from build123d import *

# Parameters (mm, degrees)
BOX001_W          = 10
BOX001_H          = 10
BOX001_DEPTH      = 8
CYLINDER_R        = 2.7
CYLINDER_DEPTH    = 10
CYLINDER001_R     = 3.5
CYLINDER001_DEPTH = 10
BOX_W             = 16
BOX_H             = 16
BOX_DEPTH         = 10


with BuildPart() as cube001:
    # Box001 → Box001 (new body)
    with BuildSketch(Plane(origin=(-5, -5, 0), x_dir=(1, 0, 0), z_dir=(0, 0, 1))):
        with Locations((5, 5)):
            Rectangle(BOX001_W, BOX001_H)
    extrude(amount=BOX001_DEPTH)


with BuildPart() as cylinder:
    # Cylinder → Cylinder (new body)
    with BuildSketch(Plane.XY.offset(10)):
        Circle(CYLINDER_R)
    extrude(amount=CYLINDER_DEPTH)


with BuildPart() as cut:
    # Cylinder001 → Cylinder001 (new body)
    with BuildSketch(Plane.XY.offset(10)):
        Circle(CYLINDER001_R)
    extrude(amount=CYLINDER001_DEPTH)

    # Cut: cut Cylinder
    add(cylinder.part, mode=Mode.SUBTRACT)


with BuildPart() as cut001:
    # Box → Box (new body)
    with BuildSketch(Plane(origin=(-8, -8, 0), x_dir=(1, 0, 0), z_dir=(0, 0, 1))):
        with Locations((8, 8)):
            Rectangle(BOX_W, BOX_H)
    extrude(amount=BOX_DEPTH)

    # Fusion: union Cut
    add(cut.part)

    # Cut001: cut Cube001
    add(cube001.part, mode=Mode.SUBTRACT)


solid = cut001.part
The model under review builds one solid part; all positions refer to its coordinate system, in mm. A direction names the side the tool comes from. Round coordinates to 2 decimals unless told otherwise and drop trailing zeros. Loops run counter-clockwise (first coordinate to the right, second up) from the corner with the lowest first, then second, coordinate; pieces in that order, holes last. Notation, with made-up numbers: (-14, 72) -> (41, 72) arc R17 cw to (41, 97) -> close; hole circle Ø9 at (44, 12.25). An arc over 180 degrees is marked (long way). Return JSON: item names as keys, results as strings.
(1) Add section B-B on x = 0. Write out the cut boundary in (y, z).
Solved:
{"outline": "(-8, 0) -> (-5, 0) -> (-5, 8) -> (5, 8) -> (5, 0) -> (8, 0) -> (8, 10) -> (3.5, 10) -> (3.5, 20) -> (2.7, 20) -> (2.7, 10) -> (-2.7, 10) -> (-2.7, 20) -> (-3.5, 20) -> (-3.5, 10) -> (-8, 10) -> close"}
(2) For faces 1 (the flat face through (-0.1, 5.4, 0)), 2 (the flat face through (-5, 0, 4)), 3 (the flat face through (-4, 0, 10)), list the 3-axis set-ups (+Z, -Z, +X, -X, +Y, -Y) from which the entire face can be reached by the end or side of a thin tool; tool diameter is ignored.
Solved:
{"face 1": "-Z, +X, -X, +Y, -Y", "face 2": "-Z", "face 3": "+Z"}
(3) Add section D-D on x = -3. Write out the cut boundary in (y, z), plus the area to 3 significant figures.
Solved:
{"outline": "(-8, 0) -> (-5, 0) -> (-5, 8) -> (5, 8) -> (5, 0) -> (8, 0) -> (8, 10) -> (1.8, 10) -> (1.8, 20) -> (-1.8, 20) -> (-1.8, 10) -> (-8, 10) -> close", "area": "116 mm2"}
(4) Add section C-C on y = -2. Write out the cut boundary in (x, z), plus the area to 3 significant figures.
Solved:
{"outline": "(-8, 0) -> (-5, 0) -> (-5, 8) -> (5, 8) -> (5, 0) -> (8, 0) -> (8, 10) -> (2.87, 10) -> (2.87, 20) -> (1.81, 20) -> (1.81, 10) -> (-1.81, 10) -> (-1.81, 20) -> (-2.87, 20) -> (-2.87, 10) -> (-8, 10) -> close", "area": "101 mm2"}
(5) For line 1 (X direction, y = 0.25, z = 1); line 2 (Y direction, x = 0, z = 12.25), list the stretches that pass through material, from the lowest coordinate up.
Solved:
{"line 1": "-8 to -5, 5 to 8", "line 2": "-3.5 to -2.7, 2.7 to 3.5"}
(6) The part is to be moulded in two halves that separate along Y. For faces 4 (the flat face through (0, -8, 5)), 5 (the flat face through (-8, 0, 5)), 6 (the flat face through (0, 5, 4)), say which applies: released by +Y, released by -Y, zero draft, split by the parting line, or undercut.
Solved:
{"face 4": "released by -Y", "face 5": "zero draft", "face 6": "undercut"}
(7) For pin 1 (4.5 mm diameter, centred on x = 0, y = 0, fed in from -Z); pin 2 (1.6 mm diameter, centred on x = 0, y = 0.5, fed in from +Z); pin 3 (3 mm diameter, centred on x = 3.5, z = 14, fed in from +Y), all flat-tipped, find the tip position at first contact; note any pin that passes through.
Solved:
{"pin 1": "z = 8", "pin 2": "z = 10", "pin 3": "y = 2.87"}
(8) Add section A-A on z = 5.75. Write out the cut boundary in (x, y), plus the area to 3 significant figures.
Solved:
{"outline": "(-8, -8) -> (8, -8) -> (8, 8) -> (-8, 8) -> close; hole (-5, -5) -> (5, -5) -> (5, 5) -> (-5, 5) -> close", "area": "156 mm2"}
